Input: part model. Units: mm. Frame: model coordinates. Coordinates: 2 decimals unless noted, no trailing zeros. Order: outer loops, then holes, each group sorted by start corner. A loop starts at its lowest first (then second) coordinate and runs counter-clockwise, first axis right, second up. Notation, with made-up numbers: (80.5, -1) - (113.5, -1) arc R16 ccw to (113.5, 22) - close; hole circle Ø2 at (88, 12.5). An arc over 180 degrees is marked (long way). One line per question, with ' | ' between items.
from build123d import *

# Parameters (mm, degrees)
SKETCH1_R           = 10
BOSS_EXTRUDE1_DEPTH = 10
BOSS_EXTRUDE1_TAPER = 3
DOME1_FACE_RADIUS   = 10
DOME1_HEIGHT        = 3
FILLET1_R           = 1


with BuildPart() as part:
    # Sketch1 → Boss-Extrude1 (new body)
    with BuildSketch(Plane(origin=(0, 0, 0), x_dir=(1, 0, 0), z_dir=(0, 1, 0))):
        Circle(SKETCH1_R)
    extrude(amount=BOSS_EXTRUDE1_DEPTH, taper=BOSS_EXTRUDE1_TAPER)

    # Dome1: a dome of height H over a round flat face of radius A is a cap of a sphere of radius (A * A + H * H) / (2 * H)
    dome1_r = (DOME1_FACE_RADIUS * DOME1_FACE_RADIUS + DOME1_HEIGHT * DOME1_HEIGHT) / (2 * DOME1_HEIGHT)
    dome1_base = Plane((0, 0, 0), z_dir=(0, -1, 0))
    with Locations(dome1_base.offset(DOME1_HEIGHT - dome1_r)):
        dome1_ball = Sphere(dome1_r, mode=Mode.PRIVATE)
    add(split(dome1_ball, bisect_by=dome1_base, keep=Keep.TOP, mode=Mode.PRIVATE))

    # Fillet1
    fillet1_edges = [part.edges().sort_by_distance(p)[0] for p in [
        (-9.475922207, 10, 0),
    ]]
    fillet(fillet1_edges, radius=FILLET1_R)


solid = part.part
Item 1: Section C-C on y = 1.25. Return the cut outline in (x, z).
Data:
outline: circle Ø19.87 at (0, 0)
Item 2: Section A-A on x = 0. Return the cut outline in (y, z).
Data:
outline: (0, -10) - (9.05, -9.53) arc R1 ccw to (10, -8.53) - (10, 8.53) arc R1 ccw to (9.05, 9.53) - (0, 10) arc R18.17 ccw to start
Item 3: Contact query for flat-ended pins moving along their axis: P1, Ø4, axis at y = 2, z = -5, coming from the +X side; P2, Ø3, axis at x = 6.5, y = 5.5, coming from the -Z side; P3, Ø12, axis at x = -4, z = -2.5, coming from the -Y side; P4, Ø1, axis at x = -3.5, y = 6, coming from the +Z side. Output: stop coordinate, or through.
Data:
P1: x = 9.44 | P2: z = -8.33 | P3: y = -3 | P4: z = 9.21
Item 4: Ray query, line 1 (X direction, y = 7.5, z = -1.25); line 2 (Z direction, x = -8, y = 7.5); line 3 (X direction, y = 8.75, z = 3.75). Return the intervals inside material, ascending.
Data:
line 1: -9.53 to 9.53 | line 2: -5.32 to 5.32 | line 3: -8.77 to 8.77
Item 5: Section B-B on y = 7. Return the cut outline in (x, z), and give its area (3 significant figures).
Data:
outline: circle Ø19.27 at (0, 0) | area: 292 mm^2
